Study the drawing (mm; zero at the part's minimum x, y, z) and answer. Give positions to 0.01 mm unless a question says otherwise; leave off trailing zeros. Write each loop counter-clockwise with the first axis right and the second up, starting at its lowest first coordinate (ties: lowest second). Pieces come first, ordered by that corner, then holes.
1) Find section D-D (z = 2.55). Determine the outline of the cut face in (x, y), plus the area to 3 significant figures.
2) Find section B-B (y = 25). Determine the outline of the cut face in (x, z).
3) Given pin 1 Ø1.8 at (x, y) = (45, 25) entering from -Z; pin 2 Ø1 at (y, z) = (27, 3.5) entering from -X; pin 3 Ø2 at (x, z) = (20.5, 3) entering from +Y; pin 4 Ø3 at (x, y) = (14, 39.5) entering from -Z, each flat-ended and moving along its own axis, determine where each tip first touches the part or whether it passes through.
4) Find section A-A (x = 5). Determine the outline of the cut face in (y, z).
5) Straight lines are drawn through the part: probe 1 along Y at (x, z) = (25, 2.2); probe 2 along X at (y, z) = (45, 1.55). For each, find the intervals that lie inside material, in ascending order.
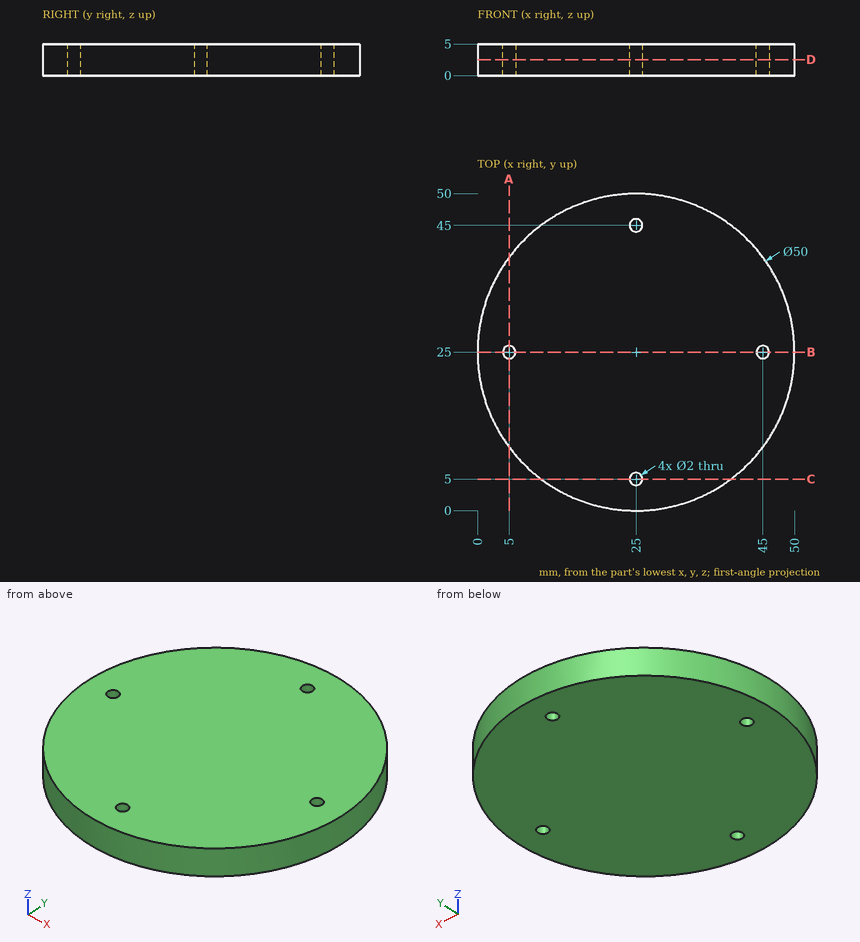
Results:
1. outline: circle Ø50 at (25, 25); hole circle Ø2 at (5, 25); hole circle Ø2 at (25, 5); hole circle Ø2 at (25, 45); hole circle Ø2 at (45, 25)
1. area: 1,950 mm2
2. outline: (0, 0) - (4, 0) - (4, 5) - (0, 5) - close; (6, 0) - (44, 0) - (44, 5) - (6, 5) - close; (46, 0) - (50, 0) - (50, 5) - (46, 5) - close
3. pin 1: passes through
3. pin 2: stops at x = 0.05
3. pin 3: stops at y = 49.75
3. pin 4: stops at z = 0
4. outline: (10, 0) - (24, 0) - (24, 5) - (10, 5) - close; (26, 0) - (40, 0) - (40, 5) - (26, 5) - close
5. probe 1: y = 0 to 4, 6 to 44, 46 to 50
5. probe 2: x = 10 to 24, 26 to 40
